Part model, mm, in its own coordinate system. A direction names the side the tool comes from. Round coordinates to 2 decimals unless told otherwise and drop trailing zeros. Write each loop counter-clockwise with the first axis right and the second up, starting at its lowest first coordinate (ties: lowest second). Pieces come first, ordered by that corner, then holes.
```python
from build123d import *

# Parameters (mm, degrees)
SKETCH1_W           = 89.63
SKETCH1_H           = 107.7
BOSS_EXTRUDE1_DEPTH = 6.35
SKETCH2_R           = 3.5
BOSS_EXTRUDE2_DEPTH = 6.35


with BuildPart() as part:
    # Sketch1 → Boss-Extrude1 (new body)
    with BuildSketch(Plane(origin=(0, 0, 0), x_dir=(1, 0, 0), z_dir=(0, 1, 0))):
        Rectangle(SKETCH1_W, SKETCH1_H)
    extrude(amount=BOSS_EXTRUDE1_DEPTH)

    # Sketch2 → Boss-Extrude2 (add)
    # profile 1 of 2: a face of its own
    with BuildSketch(Plane(origin=(0, 0, 0), x_dir=(1, 0, 0), z_dir=(0, 1, 0))):
        with BuildLine():
            Line((-40, -53.85), (-10, -53.85))
            ThreePointArc((-10, -53.85), (-15.656854249, -56.193145751), (-18, -61.85))
            ThreePointArc((-18, -61.85), (-25, -68.85), (-32, -61.85))
            ThreePointArc((-32, -61.85), (-34.343145751, -56.193145751), (-40, -53.85))
        make_face()
        with Locations(Location((-25, -61.85, 0), (0, 0, 270))):
            Circle(SKETCH2_R, mode=Mode.SUBTRACT)
    # profile 2 of 2: a face of its own
    with BuildSketch(Plane(origin=(0, 0, 0), x_dir=(1, 0, 0), z_dir=(0, 1, 0))):
        with BuildLine():
            Line((40, -53.85), (10, -53.85))
            ThreePointArc((10, -53.85), (15.656854249, -56.193145751), (18, -61.85))
            ThreePointArc((18, -61.85), (25, -68.85), (32, -61.85))
            ThreePointArc((32, -61.85), (34.343145751, -56.193145751), (40, -53.85))
        make_face()
        with Locations(Location((25, -61.85, 0), (0, 0, 270))):
            Circle(SKETCH2_R, mode=Mode.SUBTRACT)
    extrude(amount=BOSS_EXTRUDE2_DEPTH)


solid = part.part
```
Q1. Cut at C-C on x = 8. Write the cut outline in (y, z), plus the area to 3 significant figures.
Values follow:
outline: (0, -53.85) - (6.35, -53.85) - (6.35, 53.85) - (0, 53.85) - close
area: 684 mm2
Q2. Cut at B-B on y = 2.25. Write the cut outline in (x, z) (3 decimals), plus the area to 3 significant figures.
Values follow:
outline: (-44.815, -53.85) - (44.815, -53.85) - (44.815, 53.85) - (40, 53.85) arc R8 cw to (32, 61.85) arc R7 ccw to (18, 61.85) arc R8 cw to (10, 53.85) - (-10, 53.85) arc R8 cw to (-18, 61.85) arc R7 ccw to (-32, 61.85) arc R8 cw to (-40, 53.85) - (-44.815, 53.85) - close; hole circle Ø7 at (-25, 61.85); hole circle Ø7 at (25, 61.85)
area: 10,000 mm2
Q3. Which spindle directions (+Z, -Z, +X, -X, +Y, -Y) get a long thin tool onto all of the face, cutting with end or side? Do faces 1 (the flat face through (-42, 3, 53.85)), 2 (the flat face through (42, 3, 53.85)), 3 (the flat face through (-1, 3, -53.85)), 4 (the flat face through (0, 3, 53.85)), 5 (the flat face through (-44.815, 3, 1)). Say none if no direction does.
Values follow:
face 1: +Z, -X, +Y, -Y
face 2: +Z, +X, +Y, -Y
face 3: -Z, +X, -X, +Y, -Y
face 4: +Z, +Y, -Y
face 5: +Z, -Z, -X, +Y, -Y
Q4. Wall check: L1, parallel to X at y = 4, z = 61.85; L2, parallel to Z at x = -41, y = 1.5; L3, parallel to Z at x = -39.5, y = 1.75. Give the ranges that are in metal, low to high.
Values follow:
L1: x = -32 to -28.5, -21.5 to -18, 18 to 21.5, 28.5 to 32
L2: z = -53.85 to 53.85
L3: z = -53.85 to 53.87
Q5. Mould opens along Z. For faces 6 (the cylindrical face through (-34.281, 3.131, 56.256)), 7 (the cylindrical face through (-23.95, 3.13, 65.19)), 8 (the flat face through (44.815, 3, 1)), 9 (the cylindrical face through (26.05, 3.13, 65.19)) say: +Z half, -Z half, draft (parallel to the pull), parting line (faces both ways), or undercut.
Values follow:
face 6: +Z half
face 7: undercut
face 8: draft
face 9: undercut
Q6. Drop a flat-ended pin along its axis: pin 1 (2.5 mm diameter, centred on x = -43.5, y = 3.5, fed in from +Z). Give the stop position or say it passes through.
Values follow:
pin 1: stops at z = 53.85
Q7. Cut at A-A on x = 25. Write the cut outline in (y, z).
Values follow:
outline: (0, -53.85) - (6.35, -53.85) - (6.35, 58.35) - (0, 58.35) - close; (0, 65.35) - (6.35, 65.35) - (6.35, 68.85) - (0, 68.85) - close
